Input: part model. Units: mm. Frame: model coordinates. A direction names the side the tool comes from. Coordinates: 2 decimals unless noted, no trailing zeros. Loops run counter-clockwise (first coordinate to the right, second up) from the corner with the lowest first, then second, coordinate; pieces in that order, holes last.
Item 1: Pull-direction query (Y, two-part tool) for faces 3 (the flat face through (-16, 9.252, 26)), 4 (the flat face through (-16, 13.252, 27)), 5 (the cylindrical face through (-18.1, 2.7, 32.1)), 6 (the flat face through (-14.8, 4.852, 28.9)); classes: released by +Y, released by -Y, zero draft, split by the parting line, or undercut.
Item 2: Section C-C on z = 3.5. Return loops of the section in (x, y), and give its area (3 significant figures).
Item 3: Section A-A on x = -22. Return loops of the section in (y, z).
Item 4: Reachability of faces 1 (the cylindrical face through (-14.98, 2.78, 31.01)), 2 (the flat face through (-16, 9.052, 28)) from +Z, -Z, +X, -X, +Y, -Y: full face, straight path, thin tool, end or side. Return the list, or none.
Item 5: Section B-B on y = 12. Return loops of the section in (x, z).
Item 6: Contact query for flat-ended pins moving along their axis: P1, Ø5.5, axis at x = -16.5, z = 29.5, coming from the +Y side; P2, Ø5, axis at x = -18, z = 27.5, coming from the -Y side; P3, Ø1, axis at x = -19, z = 11.5, coming from the -Y side. Output: stop coordinate, or through.
Item 7: Ray query, line 1 along Z through (x, y) = (-16, 1.25); line 2 along Y through (x, z) = (-14, 25.5); line 3 along Y through (x, z) = (-14.5, 13.5). Return the intervals inside material, ascending.
```python
from build123d import *

# Parameters (mm, degrees)
F0_R         = 6.95
F1_DEPTH     = 23
F2_W         = 2.9347061182
F2_H         = 4
F3_DEPTH     = 10
F4_T1_DEPTH  = 19
F4_T3_DEPTH  = 19
F5_T4_DEPTH  = 4
F5_S5_R      = 6.95
F5_T6_DEPTH  = 7
F5_T10_DEPTH = 4
F5_S11_R     = 6.95
F5_T12_DEPTH = 7
F5_T16_DEPTH = 4
F5_S17_R     = 6.95
F5_T18_DEPTH = 7
F5_T22_DEPTH = 4
F5_S23_R     = 6.95
F5_T24_DEPTH = 7
F6_R         = 4.25
F7_DEPTH     = 15
F8_R         = 4
F10_R        = 2.5
F11_DEPTH    = 0.2
F12_R        = 2.5
F13_DEPTH    = 0.2
F9_R         = 1.5
F14_DEPTH    = 13.2510001


# Not quite as in the source:
# - a fillet or chamfer that OpenCascade refuses, or shapes differently, is made with other operations: its cross-section is extruded or revolved along the edge and cut away or added


with BuildPart() as f1:
    # F0 (on Top) → F1 (new body)
    with BuildSketch(Plane.XY):
        with Locations((-16.023524542, 6.9519880981)):
            Circle(F0_R)
    extrude(amount=F1_DEPTH)

    # F2 (on face) → F3 (join)
    with BuildSketch(Plane.XY.offset(23)):
        with Locations((-17.490877601, 11.2519880981)):
            Rectangle(F2_W, F2_H)
        with Locations((-14.5561714829, 11.2519880981)):
            Rectangle(F2_W, F2_H)
        with Locations((-17.490877601, 2.6519880981)):
            Rectangle(F2_W, F2_H)
        with Locations((-14.5561714829, 2.6519880981)):
            Rectangle(F2_W, F2_H)
    extrude(amount=F3_DEPTH)

    # F4: fillet of radius 3 on 4 edges, made by hand

    # F4_s2 → F4_t1 (cut)
    with BuildSketch(Plane.XZ.offset(-12.1519880981)):
        with BuildLine():
            ThreePointArc((-13.0888184238, 30), (-13.9674980802, 32.1213203436), (-16.0888184238, 33))
            Line((-16.0888184238, 33), (-13.0888184238, 33))
            Line((-13.0888184238, 33), (-13.0888184238, 30))
        make_face()
        with BuildLine():
            ThreePointArc((-18.9582306601, 30), (-18.0795510037, 32.1213203436), (-15.9582306601, 33))
            Line((-15.9582306601, 33), (-18.9582306601, 33))
            Line((-18.9582306601, 33), (-18.9582306601, 30))
        make_face()
    extrude(amount=F4_T1_DEPTH, mode=Mode.SUBTRACT)

    # F4_s4 → F4_t3 (cut)
    with BuildSketch(Plane.XZ.offset(-20.7519880981)):
        with BuildLine():
            ThreePointArc((-13.0888184238, 30), (-13.9674980802, 32.1213203436), (-16.0888184238, 33))
            Line((-16.0888184238, 33), (-13.0888184238, 33))
            Line((-13.0888184238, 33), (-13.0888184238, 30))
        make_face()
        with BuildLine():
            ThreePointArc((-18.9582306601, 30), (-18.0795510037, 32.1213203436), (-15.9582306601, 33))
            Line((-15.9582306601, 33), (-18.9582306601, 33))
            Line((-18.9582306601, 33), (-18.9582306601, 30))
        make_face()
    extrude(amount=F4_T3_DEPTH, mode=Mode.SUBTRACT)

    # F5: fillet of radius 7 on 4 edges, made by hand


with BuildPart() as f5_tool2:
    # F5_s3 → F5_t4 (new body)
    with BuildSketch(Plane.XZ.offset(-0.6519880981)):
        with BuildLine():
            ThreePointArc((-13.0888184238, 30), (-11.0385658921, 25.0502525317), (-6.0888184238, 23))
            Line((-6.0888184238, 23), (-6.0888184238, 22.86))
            Line((-6.0888184238, 22.86), (-13.2288184238, 22.86))
            Line((-13.2288184238, 22.86), (-13.2288184238, 30))
            Line((-13.2288184238, 30), (-13.0888184238, 30))
        make_face()
    extrude(amount=-F5_T4_DEPTH)

    # F5_s5 → F5_t6 (intersect, symmetric)
    with BuildSketch(Plane.XY.offset(26.4)):
        with Locations((-16.023524542, 6.9519880981)):
            Circle(F5_S5_R)
    extrude(amount=F5_T6_DEPTH, both=True, mode=Mode.INTERSECT)


with BuildPart() as f1_1:
    add(f1.part)

    # F5_t1: union F5_tool2
    add(f5_tool2.part)


with BuildPart() as f5_tool8:
    # F5_s9 → F5_t10 (new body)
    with BuildSketch(Plane.XZ.offset(-9.2519880981)):
        with BuildLine():
            ThreePointArc((-13.0888184238, 30), (-11.0385658921, 25.0502525317), (-6.0888184238, 23))
            Line((-6.0888184238, 23), (-6.0888184238, 22.86))
            Line((-6.0888184238, 22.86), (-13.2288184238, 22.86))
            Line((-13.2288184238, 22.86), (-13.2288184238, 30))
            Line((-13.2288184238, 30), (-13.0888184238, 30))
        make_face()
    extrude(amount=-F5_T10_DEPTH)

    # F5_s11 → F5_t12 (intersect, symmetric)
    with BuildSketch(Plane.XY.offset(26.4)):
        with Locations((-16.023524542, 6.9519880981)):
            Circle(F5_S11_R)
    extrude(amount=F5_T12_DEPTH, both=True, mode=Mode.INTERSECT)


with BuildPart() as f1_2:
    add(f1_1.part)

    # F5_t7: union F5_tool8
    add(f5_tool8.part)


with BuildPart() as f5_tool14:
    # F5_s15 → F5_t16 (new body)
    with BuildSketch(Plane.XZ.offset(-13.2519880981)):
        with BuildLine():
            ThreePointArc((-18.9582306601, 30), (-21.0084831918, 25.0502525317), (-25.9582306601, 23))
            Line((-25.9582306601, 23), (-25.9582306601, 22.86))
            Line((-25.9582306601, 22.86), (-18.8182306601, 22.86))
            Line((-18.8182306601, 22.86), (-18.8182306601, 30))
            Line((-18.8182306601, 30), (-18.9582306601, 30))
        make_face()
    extrude(amount=F5_T16_DEPTH)

    # F5_s17 → F5_t18 (intersect, symmetric)
    with BuildSketch(Plane.XY.offset(26.4)):
        with Locations((-16.023524542, 6.9519880981)):
            Circle(F5_S17_R)
    extrude(amount=F5_T18_DEPTH, both=True, mode=Mode.INTERSECT)


with BuildPart() as f1_3:
    add(f1_2.part)

    # F5_t13: union F5_tool14
    add(f5_tool14.part)


with BuildPart() as f5_tool20:
    # F5_s21 → F5_t22 (new body)
    with BuildSketch(Plane.XZ.offset(-4.6519880981)):
        with BuildLine():
            ThreePointArc((-18.9582306601, 30), (-21.0084831918, 25.0502525317), (-25.9582306601, 23))
            Line((-25.9582306601, 23), (-25.9582306601, 22.86))
            Line((-25.9582306601, 22.86), (-18.8182306601, 22.86))
            Line((-18.8182306601, 22.86), (-18.8182306601, 30))
            Line((-18.8182306601, 30), (-18.9582306601, 30))
        make_face()
    extrude(amount=F5_T22_DEPTH)

    # F5_s23 → F5_t24 (intersect, symmetric)
    with BuildSketch(Plane.XY.offset(26.4)):
        with Locations((-16.023524542, 6.9519880981)):
            Circle(F5_S23_R)
    extrude(amount=F5_T24_DEPTH, both=True, mode=Mode.INTERSECT)


with BuildPart() as f1_4:
    add(f1_3.part)

    # F5_t19: union F5_tool20
    add(f5_tool20.part)

    # F6 (on face) → F7 (cut)
    with BuildSketch(Plane(origin=(0, 0, 0), x_dir=(1, 0, 0), z_dir=(0, 0, -1))):
        with Locations((-16.023524542, -6.9519880981)):
            Circle(F6_R)
    extrude(amount=-F7_DEPTH, mode=Mode.SUBTRACT)

    # F8
    f8_edges = [f1_4.edges().sort_by_distance(p)[0] for p in [
        (-20.273525, 6.951988, 15),
    ]]
    fillet(f8_edges, radius=F8_R)

    # F10 (on face) → F11 (join)
    with BuildSketch(Plane(origin=(0, 4.6519880981, 0), x_dir=(-1, 0, 0), z_dir=(0, 1, 0))):
        with Locations((15.9582306601, 30)):
            Circle(F10_R)
    extrude(amount=F11_DEPTH)

    # F12 (on face) → F13 (join)
    with BuildSketch(Plane.XZ.offset(-9.2519880981)):
        with Locations((-16.0888184238, 30)):
            Circle(F12_R)
    extrude(amount=F13_DEPTH)

    # F9 (on face) → F14 (cut, through all)
    with BuildSketch(Plane(origin=(0, 13.2519880981, 0), x_dir=(-1, 0, 0), z_dir=(0, 1, 0))):
        with Locations((16.0888184238, 30)):
            Circle(F9_R)
    extrude(amount=-F14_DEPTH, mode=Mode.SUBTRACT)


solid = f1_4.part
```
Results found:
1. face 3: undercut
1. face 4: released by +Y
1. face 5: zero draft
1. face 6: undercut
2. outline: circle Ø13.9 at (-16.02, 6.95); hole circle Ø8.5 at (-16.02, 6.95)
2. area: 95.0 mm2
3. outline: (3.4, 0) - (10.5, 0) - (10.5, 24.23) - (9.25, 24.23) - (9.25, 23) - (4.65, 23) - (4.65, 24.23) - (3.4, 24.23) - close
4. face 1: +Y, -Y
4. face 2: +Z, +X, -X
5. outline: (-20.8, 0) - (-11.25, 0) - (-11.25, 25.27) arc R7 cw to (-13.09, 30) arc R3 ccw to (-16.02, 33) arc R3 ccw to (-18.96, 30) arc R7 cw to (-20.8, 25.27) - close; hole circle Ø3 at (-16.09, 30)
6. P1: stops at y = 13.25
6. P2: stops at y = 0.65
6. P3: stops at y = 0.46
7. line 1: z = 0 to 28.5, 31.5 to 33
7. line 2: y = 0.65 to 4.65, 9.25 to 13.25
7. line 3: y = 0.17 to 3.94, 9.96 to 13.73
